Part model, mm, in its own coordinate system. Face numbers are marked on the shaded views. A direction names the side the tool comes from. Round coordinates to 2 decimals unless told otherwise and drop trailing zeros. Loops run counter-clockwise (first coordinate to the right, second up) from the corner with the lowest first, then second, coordinate; pieces in that order, holes last.
(1) Probe probe 1 along Z at (x, y) = (0.5, 21); probe 2 along Z at (x, y) = (-6.25, 85); probe 3 along X at (y, z) = (53, -5.5). List the from-to ranges inside material, lowest first.
(2) Cut at C-C on x = -9. List the corners of the cut face in (y, z), then the cut area to 3 significant figures.
(3) Cut at A-A on y = 66. List the corners of the cut face in (x, z).
(4) Tool access for the marked faces 1 and 2: list every direction of +Z, -Z, +X, -X, +Y, -Y with a clear straight run to the whole face (end or side of a thin tool).
(5) Cut at D-D on x = -13.5. List the corners of the cut face in (y, z), then the cut area to 3 significant figures.
(6) Flat gauge pins, fed straight in: pin 1 (1 mm diameter, centred on x = -9.5, y = 80.5, fed in from +Z); pin 2 (10 mm diameter, centred on y = 74.5, z = -9.5, fed in from -X). Where does each tip first touch, or does it go through?
(7) Mould opens along Z. For the marked faces 3, 4 and 5 say: +Z half, -Z half, draft (parallel to the pull), parting line (faces both ways), or undercut.
(8) Cut at B-B on z = -4.5. List the corners of the cut face in (x, y).
Autodesk Inventor part; units mm, degrees
ref_plane "YZ Plane" through (0, 0, 0) normal (1, 0, 0) x (0, 1, 0)
ref_plane "XZ Plane" through (0, 0, 0) normal (0, 1, 0) x (-1, 0, 0)
ref_plane "XY Plane" through (0, 0, 0) normal (0, 0, 1) x (1, 0, 0)
sketch "Sketch1" plane through (0, 0, 0) normal (0, 1, 0) x (-1, 0, 0)
  line L0 (-5, 20) -> (5, 20)
  line L1 (5, 20) -> (5, -20) construction
  line L2 (5, -20) -> (-5, -20)
  line L3 (-5, -20) -> (-5, 20)
  line L4 (-5, 20) -> (5, -20) construction
  line L5 (5, 20) -> (-5, -20) construction
  arc A0 (5, -20) -> (5, 20) centre (-10, 0) ccw
  line L6 (-2.5, -17.5) -> (4.1421, -17.5)
  arc A1 (4.1421, -17.5) -> (4.1421, 17.5) centre (-10, 0) ccw
  line L7 (4.1421, 17.5) -> (-2.5, 17.5)
  line L8 (-2.5, 17.5) -> (-2.5, -17.5)
  point P0 (0, 0)
  dimension "d0" = 25
  dimension "d1" = 10
  dimension "d3" = 40
  dimension "d7" = 2.5
extrude "Extrusion1" add sketch "Sketch1" along normal blind 100
properties part number "Sanding Block"
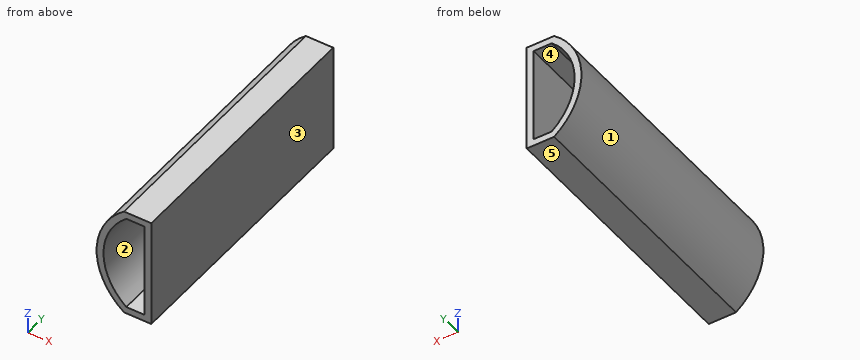
Final values:
1. probe 1: z = -20 to -17.5, 17.5 to 20
1. probe 2: z = -19 to -15.56, 15.56 to 19
1. probe 3: x = -14.39 to -11.82, 2.5 to 5
2. outline: (0, -16.25) - (100, -16.25) - (100, -12.05) - (0, -12.05) - close; (0, 12.05) - (100, 12.05) - (100, 16.25) - (0, 16.25) - close
2. area: 839 mm2
3. outline: (-5, -20) - (5, -20) - (5, 20) - (-5, 20) arc R25 ccw to start; hole (-4.14, -17.5) - (2.5, -17.5) - (2.5, 17.5) - (-4.14, 17.5) arc R22.5 ccw to start
4. face 1: -X, +Y, -Y
4. face 2: +Y, -Y
5. outline: (0, -8.53) - (100, -8.53) - (100, 8.53) - (0, 8.53) - close
5. area: 1,710 mm2
6. pin 1: stops at z = 16.25
6. pin 2: stops at x = -14.59
7. face 3: draft
7. face 4: undercut
7. face 5: -Z half
8. outline: (-14.59, 0) - (-12.05, 0) - (-12.05, 100) - (-14.59, 100) - close; (2.5, 0) - (5, 0) - (5, 100) - (2.5, 100) - close
